Design review of the part built by this model. Coordinates are the model's own, in mm. A direction names the side the tool comes from. Give positions to 0.01 mm unless a question says otherwise; leave off trailing zeros. Loops run counter-clockwise (first coordinate to the right, second up) from the corner with the lowest first, then second, coordinate; pieces in that order, holes last. Notation, with made-up numbers: (62.5, 32) - (91.5, 32) arc R17 ccw to (91.5, 60) - close; hole circle Ø9 at (9, 86). An arc over 180 degrees is marked (long way). Write each question's results on one line, items separated by ' | '.
Autodesk Inventor part; units mm, degrees
ref_plane "Work Plane3" through (0, 6.985, 0) normal (0, -1, 0) x (1, 0, 0)
ref_plane "YZ Plane" through (0, 0, 0) normal (1, 0, 0) x (0, 1, 0)
ref_plane "XZ Plane" through (0, 0, 0) normal (0, 1, 0) x (-1, 0, 0)
sketch "Sketch1" plane through (0, 0, 0) normal (0, 0, 1) x (1, 0, 0)
  line L0 (0, 6.831) -> (0, 0)
  line L1 (0, 0) -> (10.795, 0)
  line L2 (10.795, 0) -> (10.795, 3.175)
  arc A0 (0, 6.831) -> (10.795, 3.175) centre (21.59, 52.8148) ccw
  line L3 (10.795, 3.175) -> (21.59, 3.175) construction
  line L4 (21.59, 3.175) -> (21.59, 2.0148) construction
  arc A1 (10.795, 3.175) -> (21.59, 2.0148) centre (21.59, 52.8148) ccw construction
  dimension "d0" = 50.8
  dimension "d4" = 10.795
  dimension "d12" = 3.175
  dimension "d13" = 10.795
extrude "Extrusion1" add sketch "Sketch1" along normal blind 25.4
ref_plane "Work Plane3" through (0, 6.985, 0) normal (0, -1, 0) x (1, 0, 0)
sketch "Sketch4" plane through (0, 6.985, 0) normal (0, -1, 0) x (1, 0, 0)
  line L0 (3.0162, 0) -> (3.0163, 25.4)
  line L1 (0, 25.4) -> (10.795, 25.4)
  line L2 (3.0163, 25.4) -> (7.7788, 25.4)
  line L3 (7.7788, 25.4) -> (7.7788, 23.495)
  line L4 (7.7788, 23.495) -> (10.795, 23.495)
  line L5 (10.795, 0) -> (10.795, 25.4)
  line L6 (10.795, 23.495) -> (10.795, 10.795)
  line L7 (10.795, 10.795) -> (7.7788, 10.795)
  line L8 (7.7788, 10.795) -> (7.7788, 0)
  line L9 (7.7788, 0) -> (3.0162, 0)
  line L10 (10.795, 0) -> (0, 0) construction
  point P0 (5.3975, 0)
  point P1 (5.3975, 0)
  dimension "d22" = 10.795
  dimension "d23" = 12.7
  dimension "d24" = 4.7625
extrude "Extrusion3" cut sketch "Sketch4" along normal blind 6.096 contours L0 L1 L3 L4 L5 L7 L8 L9
properties part number "WireGuideToSail2" material "ABS Plastic"
(1) Tool access review of faces 1 (the flat face through (0, 3, 13)), 2 (the flat face through (7.779, 2, 5)), 3 (the flat face through (9, 2, 23.495)): name each direction out of +Z, -Z, +X, -X, +Y, -Y from which nothing blocks a thin tool from reaching the whole face with its end or side.
Answers below:
face 1: +Z, -Z, -X, +Y, -Y | face 2: +Z, -Z, +Y | face 3: +X, +Y
(2) Draft analysis for pull direction Z (two halves, no side actions). For faces 4 (the flat face through (4.1, 0.4, 0)), 5 (the flat face through (9, 2, 10.795)), 6 (the flat face through (7.779, 2, 24)), state which applies: pulls with the +Z half, pulls with the -Z half, needs draft (parallel to the pull), parting line crosses it, or undercut.
Answers below:
face 4: pulls with the -Z half | face 5: undercut | face 6: needs draft
(3) Insertion check: P1, Ø1.5, axis at y = 5.5, z = 17, coming from the +X side; P2, Ø0.9, axis at x = 9, y = 3, coming from the -Z side; P3, Ø2.5, axis at x = 8, z = 18, coming from the +Y side. Each pin has a flat end and moves straight along its axis. Give the tip position at first contact, or say it passes through.
Answers below:
P1: x = 3.02 | P2: z = 0 | P3: y = 0.89
(4) Wall thickness on line 1 along X through (y, z) = (1.25, 3) (3 decimals); line 2 along Y through (x, z) = (4.5, 14.5); line 3 along X through (y, z) = (1.75, 23): over which ranges is each line inside the solid? List them lowest first. Write a range as from..to.
Answers below:
line 1: 0..3.016, 7.779..10.795 | line 2: 0..0.89 | line 3: 0..3.02
(5) Take a section at C-C on x = 6.5. Give the boundary of the cut face in (y, z).
Answers below:
outline: (0, 0) - (0.89, 0) - (0.89, 25.4) - (0, 25.4) - close
(6) Take a section at D-D on y = 5. Give the boundary of the cut face in (x, z), plus the area to 3 significant figures.
Answers below:
outline: (0, 0) - (3.02, 0) - (3.02, 25.4) - (0, 25.4) - close | area: 76.6 mm2
(7) Take a section at A-A on y = 1.25. Give the boundary of the cut face in (x, z) (3 decimals).
Answers below:
outline: (0, 0) - (3.016, 0) - (3.016, 25.4) - (0, 25.4) - close; (7.779, 0) - (10.795, 0) - (10.795, 10.795) - (7.779, 10.795) - close; (7.779, 23.495) - (10.795, 23.495) - (10.795, 25.4) - (7.779, 25.4) - close
(8) Take a section at B-B on z = 4.5. Give the boundary of the cut face in (x, y) (3 decimals), plus the area to 3 significant figures.
Answers below:
outline: (0, 0) - (10.795, 0) - (10.795, 3.175) arc R50.803 cw to (7.779, 3.928) - (7.779, 0.889) - (3.016, 0.889) - (3.016, 5.532) arc R50.803 cw to (0, 6.831) - close | area: 33.5 mm2
